Verification items for the finished model (mm, model axes). A direction names the side the tool comes from. Coordinates: 2 decimals unless noted, no trailing zeros. Loops run counter-clockwise (first coordinate to the right, second up) from the corner with the lowest first, then second, coordinate; pieces in that order, holes last.
Q1. Sectioned sample at B-B (z = 6.5). Enter the section's corners in (x, y).
Q2. Material ranges on probe 1 along Y at (x, z) = (0, 4.5); probe 2 along X at (y, z) = (45.5, 4); probe 3 along Y at (x, z) = (12, 3), recorded low to high.
Q3. Sectioned sample at A-A (x = 0). Enter the section's corners in (y, z).
Q4. Access from +Z, -Z, +X, -X, +Y, -Y to the whole of each face (thin tool, end or side, straight path). Record for faces 1 (the face through (11.73, 16.78, 3.94)), 2 (the face through (11.29, 44.2, 3.83)).
Q5. Mould release check, pull along Y, two halves, no side actions. Record for faces 3 (the face through (-7.25, 0.05, 3.94)), 4 (the face through (14.724, -4.521, 3.944)), 5 (the face through (10, 40.5, 4)): +Y half, -Y half, draft (parallel to the pull), parting line (faces both ways), or undercut.
Q6. Go/stop test with flat-tipped pins: P1, Ø2, axis at x = -10, z = 4, coming from the +Y side; P2, Ø8.5, axis at x = 0, y = 9, coming from the -Z side; P3, Ø3, axis at x = 30.5, z = 4.5, coming from the +Y side; P4, Ø1, axis at y = 29, z = 7, coming from the -X side. Record where each tip stops, or that it passes through.
Q7. Sectioned sample at D-D (x = 30). Enter the section's corners in (y, z).
Q8. Sectioned sample at C-C (y = 9). Enter the section's corners in (x, z), then the cut area to 3 significant figures.
```python
from build123d import *

# Parameters (mm, degrees)
SKETCH_1_R          = 1.25
SKETCH_1_R_2        = 7
EXTRUDE_1_DEPTH     = 8
SKETCH_2_R          = 1.3
CUT_EXTRUDE_1_DEPTH = 7.5
CHAMFER_1_SIZE      = 0.2


with BuildPart() as part:
    # 草圖1 → 填料-伸長1 (new body)
    with BuildSketch(Plane.XY):
        with BuildLine():
            Line((0, -5), (-13.098093889, -5))
            ThreePointArc((-13.098093889, -5), (-14.704398953, -4.533729275), (-15.811388666, -3.279856027))
            Line((-15.811388666, -3.279856027), (-40, 48))
            Line((-40, 48), (0, 48))
            Line((0, 48), (40, 48))
            Line((40, 48), (15.811388666, -3.279856027))
            ThreePointArc((15.811388666, -3.279856027), (14.704398953, -4.533729275), (13.098093889, -5))
            Line((13.098093889, -5), (0, -5))
        make_face()
        with Locations((6, 0)):
            Circle(SKETCH_1_R, mode=Mode.SUBTRACT)
        with Locations((-6, 0)):
            Circle(SKETCH_1_R, mode=Mode.SUBTRACT)
        with Locations((-12, 18)):
            Circle(SKETCH_1_R, mode=Mode.SUBTRACT)
        with Locations((12, 18)):
            Circle(SKETCH_1_R, mode=Mode.SUBTRACT)
        with Locations((0, 9)):
            Circle(SKETCH_1_R_2, mode=Mode.SUBTRACT)
    extrude(amount=EXTRUDE_1_DEPTH)

    # 草圖2 → 除料-伸長1 (cut)
    with BuildSketch(Plane(origin=(0, 48, 0), x_dir=(1, 0, 0), z_dir=(0, 1, 0))):
        with Locations(Location((-10, -4, 0), (0, 0, 270))):
            Circle(SKETCH_2_R)
        with Locations(Location((-30, -4, 0), (0, 0, 270))):
            Circle(SKETCH_2_R)
        with Locations(Location((10, -4, 0), (0, 0, 270))):
            Circle(SKETCH_2_R)
        with Locations(Location((30, -4, 0), (0, 0, 270))):
            Circle(SKETCH_2_R)
    extrude(amount=-CUT_EXTRUDE_1_DEPTH, mode=Mode.SUBTRACT)

    # 導角1
    chamfer_1_edges = [part.edges().sort_by_distance(p)[0] for p in [
        (30, 48, 2.7),
        (10, 48, 2.7),
        (-30, 48, 2.7),
        (-10, 48, 2.7),
    ]]
    chamfer(chamfer_1_edges, length=CHAMFER_1_SIZE)


solid = part.part
```
Geometry check:
1. outline: (-40, 48) - (-15.81, -3.28) arc R3 ccw to (-13.1, -5) - (13.1, -5) arc R3 ccw to (15.81, -3.28) - (40, 48) - close; hole circle Ø2.5 at (-12, 18); hole circle Ø2.5 at (-6, 0); hole circle Ø14 at (0, 9); hole circle Ø2.5 at (6, 0); hole circle Ø2.5 at (12, 18)
2. probe 1: y = -5 to 2, 16 to 48
2. probe 2: x = -38.82 to -31.3, -28.7 to -11.3, -8.7 to 8.7, 11.3 to 28.7, 31.3 to 38.82
2. probe 3: y = -5 to 16.75, 19.25 to 48
3. outline: (-5, 0) - (2, 0) - (2, 8) - (-5, 8) - close; (16, 0) - (48, 0) - (48, 8) - (16, 8) - close
4. face 1: +Z, -Z
4. face 2: +Y
5. face 3: undercut
5. face 4: -Y half
5. face 5: +Y half
6. P1: stops at y = 40.5
6. P2: passes through
6. P3: stops at y = 48
6. P4: stops at x = -31.27
7. outline: (26.8, 0) - (48, 0) - (48, 2.5) - (47.8, 2.7) - (40.5, 2.7) - (40.5, 5.3) - (47.8, 5.3) - (48, 5.5) - (48, 8) - (26.8, 8) - close
8. outline: (-21.6, 0) - (-7, 0) - (-7, 8) - (-21.6, 8) - close; (7, 0) - (21.6, 0) - (21.6, 8) - (7, 8) - close
8. area: 234 mm2
